from build123d import *

# Parameters (mm, degrees)
SKETCH_W        = 100
SKETCH_H        = 84
PAD_DEPTH       = 10
SKETCH001_R     = 2.1
POCKET_DEPTH    = 10
SKETCH002_R     = 3.2
POCKET001_DEPTH = 10
SKETCH003_R     = 4
POCKET002_DEPTH = 5
POCKET003_DEPTH = 4
POCKET004_DEPTH = 5.2
FILLET_R        = 4
CHAMFER_SIZE    = 0.4
CHAMFER001_SIZE = 0.4


with BuildPart() as part:
    # Sketch → Pad (new body)
    with BuildSketch(Plane.XY):
        with Locations((50, 42)):
            Rectangle(SKETCH_W, SKETCH_H)
    extrude(amount=PAD_DEPTH)

    # Sketch001 (on Face6 of Pad) → Pocket (cut)
    with BuildSketch(Plane.XY.offset(10)):
        with Locations((6, 78)):
            Circle(SKETCH001_R)
        with Locations((30, 78)):
            Circle(SKETCH001_R)
        with Locations((6, 60)):
            Circle(SKETCH001_R)
        with Locations((30, 60)):
            Circle(SKETCH001_R)
        with Locations((6, 24)):
            Circle(SKETCH001_R)
        with Locations((30, 24)):
            Circle(SKETCH001_R)
        with Locations((6, 6)):
            Circle(SKETCH001_R)
        with Locations((30, 6)):
            Circle(SKETCH001_R)
        with Locations((70, 78)):
            Circle(SKETCH001_R)
        with Locations((94, 78)):
            Circle(SKETCH001_R)
        with Locations((70, 60)):
            Circle(SKETCH001_R)
        with Locations((94, 60)):
            Circle(SKETCH001_R)
        with Locations((70, 24)):
            Circle(SKETCH001_R)
        with Locations((94, 24)):
            Circle(SKETCH001_R)
        with Locations((70, 6)):
            Circle(SKETCH001_R)
        with Locations((94, 6)):
            Circle(SKETCH001_R)
        with Locations((35, 47)):
            Circle(SKETCH001_R)
        with Locations((65, 47)):
            Circle(SKETCH001_R)
        with Locations((35, 37)):
            Circle(SKETCH001_R)
        with Locations((65, 37)):
            Circle(SKETCH001_R)
    extrude(amount=-POCKET_DEPTH, mode=Mode.SUBTRACT)

    # Sketch002 (on Face5 of Pocket) → Pocket001 (cut)
    with BuildSketch(Plane.XY.offset(10)):
        with Locations((20, 62)):
            Circle(SKETCH002_R)
        with Locations((20, 22)):
            Circle(SKETCH002_R)
        with Locations((80, 62)):
            Circle(SKETCH002_R)
        with Locations((80, 22)):
            Circle(SKETCH002_R)
    extrude(amount=-POCKET001_DEPTH, mode=Mode.SUBTRACT)

    # Sketch003 (on Face5 of Pocket001) → Pocket002 (cut)
    with BuildSketch(Plane.XY.offset(10)):
        with Locations((6, 78)):
            Circle(SKETCH003_R)
        with Locations((30, 78)):
            Circle(SKETCH003_R)
        with Locations((30, 60)):
            Circle(SKETCH003_R)
        with Locations((6, 60)):
            Circle(SKETCH003_R)
        with Locations((70, 78)):
            Circle(SKETCH003_R)
        with Locations((94, 78)):
            Circle(SKETCH003_R)
        with Locations((70, 60)):
            Circle(SKETCH003_R)
        with Locations((94, 60)):
            Circle(SKETCH003_R)
        with Locations((6, 24)):
            Circle(SKETCH003_R)
        with Locations((30, 24)):
            Circle(SKETCH003_R)
        with Locations((6, 6)):
            Circle(SKETCH003_R)
        with Locations((30, 6)):
            Circle(SKETCH003_R)
        with Locations((70, 24)):
            Circle(SKETCH003_R)
        with Locations((94, 24)):
            Circle(SKETCH003_R)
        with Locations((70, 6)):
            Circle(SKETCH003_R)
        with Locations((94, 6)):
            Circle(SKETCH003_R)
        with Locations((35, 47)):
            Circle(SKETCH003_R)
        with Locations((35, 37)):
            Circle(SKETCH003_R)
        with Locations((65, 37)):
            Circle(SKETCH003_R)
        with Locations((65, 47)):
            Circle(SKETCH003_R)
    extrude(amount=-POCKET002_DEPTH, mode=Mode.SUBTRACT)

    # Sketch003 (on Face5 of Pocket001) → Pocket003 (cut)
    with BuildSketch(Plane.XY.offset(10)):
        with Locations((6, 78)):
            Circle(SKETCH003_R)
        with Locations((30, 78)):
            Circle(SKETCH003_R)
        with Locations((30, 60)):
            Circle(SKETCH003_R)
        with Locations((6, 60)):
            Circle(SKETCH003_R)
        with Locations((70, 78)):
            Circle(SKETCH003_R)
        with Locations((94, 78)):
            Circle(SKETCH003_R)
        with Locations((70, 60)):
            Circle(SKETCH003_R)
        with Locations((94, 60)):
            Circle(SKETCH003_R)
        with Locations((6, 24)):
            Circle(SKETCH003_R)
        with Locations((30, 24)):
            Circle(SKETCH003_R)
        with Locations((6, 6)):
            Circle(SKETCH003_R)
        with Locations((30, 6)):
            Circle(SKETCH003_R)
        with Locations((70, 24)):
            Circle(SKETCH003_R)
        with Locations((94, 24)):
            Circle(SKETCH003_R)
        with Locations((70, 6)):
            Circle(SKETCH003_R)
        with Locations((94, 6)):
            Circle(SKETCH003_R)
        with Locations((35, 47)):
            Circle(SKETCH003_R)
        with Locations((35, 37)):
            Circle(SKETCH003_R)
        with Locations((65, 37)):
            Circle(SKETCH003_R)
        with Locations((65, 47)):
            Circle(SKETCH003_R)
    extrude(amount=-POCKET003_DEPTH, mode=Mode.SUBTRACT)

    # Sketch004 (on Face4 of Pocket003) → Pocket004 (cut)
    with BuildSketch(Plane(origin=(0, 0, 0), x_dir=(1, 0, 0), z_dir=(0, 0, -1))):
        Polygon((14.42356, -23.704889), (18.688257, -27.681783), (24.264697, -25.976895), (25.57644, -20.295111), (21.311743, -16.318217), (15.735303, -18.023105), align=None)
        Polygon((74.318217, -20.688257), (76.023105, -26.264697), (81.704889, -27.57644), (85.681783, -23.311743), (83.976895, -17.735303), (78.295111, -16.42356), align=None)
        Polygon((74.42356, -63.704889), (78.688257, -67.681783), (84.264697, -65.976895), (85.57644, -60.295111), (81.311743, -56.318217), (75.735303, -58.023105), align=None)
        Polygon((14.318217, -60.688257), (16.023105, -66.264697), (21.704889, -67.57644), (25.681783, -63.311743), (23.976895, -57.735303), (18.295111, -56.42356), align=None)
    extrude(amount=-POCKET004_DEPTH, mode=Mode.SUBTRACT)

    # Fillet
    fillet_edges = [part.edges().sort_by_distance(p)[0] for p in [
        (100, 0, 5),
        (100, 84, 5),
        (0, 0, 5),
        (0, 84, 5),
    ]]
    fillet(fillet_edges, radius=FILLET_R)

    # Chamfer
    chamfer_edges = [part.edges().sort_by_distance(p)[0] for p in [
        (50, 84, 10),
        (1.171573, 82.828427, 10),
        (98.828427, 82.828427, 10),
        (0, 42, 10),
        (100, 42, 10),
        (1.171573, 1.171573, 10),
        (98.828427, 1.171573, 10),
        (50, 0, 10),
        (90, 6, 10),
        (66, 6, 10),
        (90, 24, 10),
        (76.8, 22, 10),
        (66, 24, 10),
        (61, 37, 10),
        (26, 6, 10),
        (2, 6, 10),
        (26, 24, 10),
        (31, 37, 10),
        (16.8, 22, 10),
        (2, 24, 10),
        (90, 60, 10),
        (61, 47, 10),
        (66, 60, 10),
        (76.8, 62, 10),
        (90, 78, 10),
        (66, 78, 10),
        (31, 47, 10),
        (26, 60, 10),
        (2, 60, 10),
        (26, 78, 10),
        (16.8, 62, 10),
        (2, 78, 10),
    ]]
    chamfer(chamfer_edges, length=CHAMFER_SIZE)

    # Chamfer001
    chamfer001_edges = [part.edges().sort_by_distance(p)[0] for p in [
        (50, 84, 0),
        (1.171573, 82.828427, 0),
        (98.828427, 82.828427, 0),
        (0, 42, 0),
        (100, 42, 0),
        (1.171573, 1.171573, 0),
        (98.828427, 1.171573, 0),
        (50, 0, 0),
        (91.9, 6, 0),
        (75.170661, 23.476477, 0),
        (78.863997, 26.920569, 0),
        (83.693336, 25.444092, 0),
        (84.829339, 20.523523, 0),
        (81.136003, 17.079431, 0),
        (76.306664, 18.555908, 0),
        (67.9, 6, 0),
        (91.9, 24, 0),
        (67.9, 24, 0),
        (62.9, 37, 0),
        (27.9, 6, 0),
        (3.9, 6, 0),
        (16.555908, 25.693336, 0),
        (21.476477, 26.829339, 0),
        (24.920569, 23.136003, 0),
        (23.444092, 18.306664, 0),
        (18.523523, 17.170661, 0),
        (15.079431, 20.863997, 0),
        (27.9, 24, 0),
        (32.9, 37, 0),
        (3.9, 24, 0),
        (91.9, 60, 0),
        (62.9, 47, 0),
        (67.9, 60, 0),
        (76.555908, 65.693336, 0),
        (81.476477, 66.829339, 0),
        (84.920569, 63.136003, 0),
        (83.444092, 58.306664, 0),
        (78.523523, 57.170661, 0),
        (75.079431, 60.863997, 0),
        (91.9, 78, 0),
        (67.9, 78, 0),
        (32.9, 47, 0),
        (27.9, 60, 0),
        (3.9, 60, 0),
        (27.9, 78, 0),
        (15.170661, 63.476477, 0),
        (18.863997, 66.920569, 0),
        (23.693336, 65.444092, 0),
        (24.829339, 60.523523, 0),
        (21.136003, 57.079431, 0),
        (16.306664, 58.555908, 0),
        (3.9, 78, 0),
    ]]
    chamfer(chamfer001_edges, length=CHAMFER001_SIZE)


solid = part.part
Input: part model. Units: mm. Frame: model coordinates. A direction names the side the tool comes from. Coordinates: 2 decimals unless noted, no trailing zeros. Answer as a JSON object with one key per item and string values. Group by question number.
(1) Mould query, pull axis X, two halves, no side actions, for faces 4 (the face through (33.334, 45.722, 2.732)), 5 (the face through (49, 0, 5)). Classes: pulls with the +X half, pulls with the -X half, needs draft (parallel to the pull), parting line crosses it, or undercut.
(2) Section A-A on z = 8. Give the number of separate pieces and of enclosed holes in the cut face, plus the area to 3 significant figures.
(3) Set-up query: faces 1 (the face through (71.846, 74.451, 7.332)), 2 (the face through (28.334, 58.722, 2.732)), 3 (the face through (83.67, 25.47, 2.77)). Return all of +Z, -Z, +X, -X, +Y, -Y with unobstructed straight access to the full face (end or side cutting, diameter ignored); none if empty.
(4) Contact query for flat-ended pins moving along their axis: P1, Ø4, axis at x = 93, y = 24, coming from the +Z side; P2, Ø6.5, axis at x = 6.5, y = 5, coming from the +Z side. Output: stop coordinate, or through.
(5) Ray query, line 1 along Y through (x, z) = (30, 2.75); line 2 along Y through (x, z) = (70, 6.8); line 3 along X through (y, z) = (76, 7.75). Return the intervals inside material, ascending. Write a range as [from, to].
Result set:
{
 "1": {"face 4": "undercut", "face 5": "needs draft"},
 "2": {"separate pieces": "1", "enclosed holes": "24", "area": "7,250 mm2"},
 "3": {"face 1": "+Z", "face 2": "+Z, -Z", "face 3": "-Z"},
 "4": {"P1": "stops at z = 5", "P2": "stops at z = 9.97"},
 "5": {"line 1": "y = [0, 3.9], [8.1, 21.9], [26.1, 57.9], [62.1, 75.9], [80.1, 84]", "line 2": "y = [0, 2], [10, 20], [28, 56], [64, 74], [82, 84]", "line 3": "x = [0, 2.54], [9.46, 26.54], [33.46, 66.54], [73.46, 90.54], [97.46, 100]"}
}
